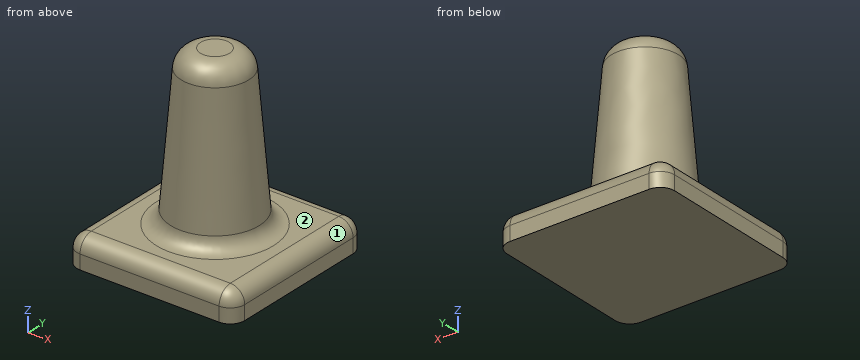
```python
from build123d import *

# Parameters (mm, degrees)
F0_W     = 35
F0_H     = 35
F0_R     = 7.96
F1_DEPTH = 6
F2_R     = 9.46
F4_R     = 6.71
F6_R     = 4
F7_R     = 3


with BuildPart() as f1:
    # F0 (on Top) → F1 (new body)
    with BuildSketch(Plane.XY):
        Rectangle(F0_W, F0_H)
        Circle(F0_R, mode=Mode.SUBTRACT)
        Circle(F0_R)
    extrude(amount=F1_DEPTH)

    # F2 (on face) → F5 section 0
    with BuildSketch(Plane.XY.offset(6)):
        Circle(F2_R)
    # F4 (on offset) → F5 section 1
    with BuildSketch(Plane.XY.offset(39)):
        Circle(F4_R)
    loft()

    # F6
    f6_edges = [f1.edges().sort_by_distance(p)[0] for p in [
        (-6.71, 0, 39),
    ]]
    fillet(f6_edges, radius=F6_R)

    # F7
    f7_edges = [f1.edges().sort_by_distance(p)[0] for p in [
        (0, 17.5, 6),
        (17.5, 0, 6),
        (-17.5, 0, 6),
        (0, -17.5, 6),
        (-9.46, 0, 6),
        (-17.5, -17.5, 3),
        (-17.5, 17.5, 3),
        (17.5, -17.5, 3),
        (17.5, 17.5, 3),
    ]]
    fillet(f7_edges, radius=F7_R)


solid = f1.part
```
Input: part model. Units: mm. Frame: model coordinates. Face numbers are marked on the shaded views. A direction names the side the tool comes from. Round coordinates to 2 decimals unless told otherwise and drop trailing zeros. Loops run counter-clockwise (first coordinate to the right, second up) from the corner with the lowest first, then second, coordinate; pieces in that order, holes last. Notation, with made-up numbers: (62, -8.75) -> (102, -8.75) arc R22 cw to (102, 28.25) -> close; hole circle Ø8 at (74, 83). An arc over 180 degrees is marked (long way). Use one line per item in the form item = value. Start each with the question number.
Item 1: Section query A-A on x = 13.5. Return the cut outline in (y, z), then the cut area to 3 significant figures.
Item 2: Set-up query: the marked faces 1 and 2. Return all of +Z, -Z, +X, -X, +Y, -Y with unobstructed straight access to the full face (end or side cutting, diameter ignored); none if empty.
Item 3: Section query C-C on z = 31. Return the cut outline in (x, y).
Item 4: Contact query for flat-ended pins moving along their axis: pin 1 Ø6 at (x, y) = (-1, 9.5) entering from +Z; pin 2 Ø2 at (y, z) = (-7.5, 18.5) entering from +X; pin 3 Ø1.5 at (y, z) = (-8, 34.5) entering from -X; pin 4 Ø1.5 at (y, z) = (7.5, 10.5) entering from +X. Output: stop coordinate, or through.
Item 5: Material intervals for L1, parallel to Z at x = 12, y = 3.5; L2, parallel to Z at x = 4, y = -4.5; L3, parallel to X at y = 0, z = 33.5, sorted ascending. Write a range as from..to.
Item 6: Section query B-B on z = 21. Return the cut outline in (x, y).
Ans:
q1.outline = (-17.5, 0) -> (17.5, 0) -> (17.5, 3) arc R3 ccw to (14.5, 6) -> (-14.5, 6) arc R3 ccw to (-17.5, 3) -> close
q1.area = 206 mm^2
q2.face_1 = +Z, +X, +Y, -Y
q2.face_2 = +Z
q3.outline = circle Ø14.75 at (0, 0)
q4.pin_1 = 36.89
q4.pin_2 = 5.36
q4.pin_3 = through
q4.pin_4 = 6.09
q5.L1 = 0..6
q5.L2 = 0..37.66
q5.L3 = -7.17..7.17
q6.outline = circle Ø16.42 at (0, 0)
